Geometry check sheet. Reference: the model listing, model coordinates, mm. A direction names the side the tool comes from. Round coordinates to 2 decimals unless told otherwise and drop trailing zeros. Order: outer loops, then holes, each group sorted by start corner. A loop starts at its lowest first (then second) coordinate and runs counter-clockwise, first axis right, second up.
(1) Sectioned sample at A-A (y = 8). Record the boundary of the cut face in (x, z), plus the area to 3 significant figures.
(2) Go/stop test with flat-tipped pins: pin 1 (5 mm diameter, centred on x = -86, y = 2.5, fed in from -Z); pin 2 (4.5 mm diameter, centred on x = 4.5, y = 6.5, fed in from -Z); pin 3 (6 mm diameter, centred on x = -130.5, y = 4, fed in from -Z); pin 4 (0.6 mm diameter, centred on x = -24, y = 0.5, fed in from +Z). Record where each tip stops, or that it passes through.
(3) Release check for a two-part mould opening along X. For faces 1 (the face through (-104.89, 6.45, -107.23)), 2 (the face through (-2.734, 10.887, -2.675)), 3 (the face through (4, 8, -91)) record: +X half, -X half, draft (parallel to the pull), parting line (faces both ways), or undercut.
(4) Material ranges on line 1 along Y through (x, z) = (-51.5, -73.5); line 2 along X through (y, z) = (2.75, -13.5); line 3 along Z through (x, y) = (-60.5, 7.25), recorded low to high.
(5) Set-up check for faces 4 (the face through (-90, 8, -5)), 5 (the face through (-103.064, 0.838, -100.822)), 6 (the face through (-1, 11.8, -2)), 7 (the face through (5, 5.65, -95)), 8 (the face through (4, 8, -99.277)): record each of +Z, -Z, +X, -X, +Y, -Y from which the full face is reachable in a straight line by a thin tool's end or side.
from build123d import *

# Parameters (mm, degrees)
SKETCH1_R           = 150
BOSS_EXTRUDE3_DEPTH = 10
CUT_EXTRUDE2_DEPTH  = 10
BOSS_EXTRUDE4_DEPTH = 1.8
SKETCH6_W           = 3
SKETCH6_H           = 7
BOSS_EXTRUDE5_DEPTH = 2
SKETCH7_W           = 7
SKETCH7_H           = 3
BOSS_EXTRUDE6_DEPTH = 2
SKETCH8_W           = 10
SKETCH8_H           = 10
CUT_EXTRUDE3_DEPTH  = 5
SKETCH9_W           = 9.193751657
SKETCH9_H           = 8.277315045
BOSS_EXTRUDE7_DEPTH = 4.35
CHAMFER1_SIZE       = 1
CUT_EXTRUDE4_DEPTH  = 1.7
CUT_EXTRUDE5_DEPTH  = 0.8
FILLET1_R           = 3
FILLET2_R           = 1.4


with BuildPart() as part:
    # Sketch1 → Boss-Extrude3 (new body)
    with BuildSketch(Plane(origin=(0, 0, 0), x_dir=(1, 0, 0), z_dir=(0, 1, 0))):
        with Locations(Location((0, 0, 0), (0, 0, 270))):
            Circle(SKETCH1_R)
    extrude(amount=BOSS_EXTRUDE3_DEPTH)

    # Sketch4 → Cut-Extrude2 (cut)
    with BuildSketch(Plane(origin=(0, 10, 0), x_dir=(1, 0, 0), z_dir=(0, 1, 0))):
        Polygon((0, 0), (0, 162.329653064), (183.678217859, 162.329653064), (183.678217859, -176.427761891), (-217.916482153, -176.427761891), (-217.916482153, 0), align=None)
    extrude(amount=-CUT_EXTRUDE2_DEPTH, mode=Mode.SUBTRACT)

    # Sketch5 → Boss-Extrude4 (add)
    with BuildSketch(Plane(origin=(0, 10, 0), x_dir=(1, 0, 0), z_dir=(0, 1, 0))):
        with BuildLine():
            Line((0, 3.825), (0, 0))
            Line((0, 0), (-3.825, 0))
            ThreePointArc((-3.825, 0), (-2.704683438, 2.704683438), (0, 3.825))
        make_face()
    extrude(amount=BOSS_EXTRUDE4_DEPTH)

    # Sketch6 → Boss-Extrude5 (add)
    with BuildSketch(Plane(origin=(0, 10, 0), x_dir=(1, 0, 0), z_dir=(0, 1, 0))):
        with Locations((-28.5, 3.5)):
            Rectangle(SKETCH6_W, SKETCH6_H)
    extrude(amount=BOSS_EXTRUDE5_DEPTH)

    # Sketch7 → Boss-Extrude6 (add)
    with BuildSketch(Plane(origin=(0, 10, 0), x_dir=(1, 0, 0), z_dir=(0, 1, 0))):
        with Locations((-3.5, 28.5)):
            Rectangle(SKETCH7_W, SKETCH7_H)
    extrude(amount=BOSS_EXTRUDE6_DEPTH)

    # Sketch8 → Cut-Extrude3 (cut)
    with BuildSketch(Plane(origin=(0, 10, 0), x_dir=(1, 0, 0), z_dir=(0, 1, 0))):
        with Locations((-95, 5)):
            Rectangle(SKETCH8_W, SKETCH8_H)
    extrude(amount=-CUT_EXTRUDE3_DEPTH, mode=Mode.SUBTRACT)

    # Sketch9 → Boss-Extrude7 (add)
    with BuildSketch(Plane(origin=(0, 10, 0), x_dir=(1, 0, 0), z_dir=(0, 1, 0))):
        with Locations((4.596875828, 95.138657523)):
            Rectangle(SKETCH9_W, SKETCH9_H)
    extrude(amount=-BOSS_EXTRUDE7_DEPTH)

    # Chamfer1
    chamfer1_edges = [part.edges().sort_by_distance(p)[0] for p in [
        (9.193751657, 7.825, -99.277315045),
        (9.193751657, 7.825, -91),
    ]]
    chamfer(chamfer1_edges, length=CHAMFER1_SIZE)

    # Sketch10 → Cut-Extrude4 (cut)
    with BuildSketch(Plane.XZ):
        with BuildLine():
            Line((-140.926536809, 0), (-144.178447036, 0))
            ThreePointArc((-144.178447036, 0), (-101.9495576, -101.9495576), (0, -144.178447036))
            Line((0, -144.178447036), (0, -140.926536809))
            ThreePointArc((0, -140.926536809), (-99.650109827, -99.650109827), (-140.926536809, 0))
        make_face()
    extrude(amount=-CUT_EXTRUDE4_DEPTH, mode=Mode.SUBTRACT)

    # Sketch11 → Cut-Extrude5 (cut)
    with BuildSketch(Plane(origin=(0, 0, 0), x_dir=(-1, 0, 0), z_dir=(0, -1, 0))):
        Polygon((47, 0), (50, 0), (50, 50), (0, 50), (0, 47), (47, 47), align=None)
    extrude(amount=-CUT_EXTRUDE5_DEPTH, mode=Mode.SUBTRACT)

    # Fillet1
    fillet1_edges = [part.edges().sort_by_distance(p)[0] for p in [
        (-106.066017178, 0, -106.066017178),
    ]]
    fillet(fillet1_edges, radius=FILLET1_R)

    # Fillet2
    fillet2_edges = [part.edges().sort_by_distance(p)[0] for p in [
        (0, 5.65, -95.138657523),
    ]]
    fillet(fillet2_edges, radius=FILLET2_R)


solid = part.part
Answer below:
1. outline: (-150, 0) arc R150 ccw to (0, -150) - (0, -99.28) - (8.19, -99.28) - (9.19, -98.28) - (9.19, -92) - (8.19, -91) - (0, -91) - (0, 0) - (-90, 0) - (-90, -10) - (-100, -10) - (-100, 0) - close
1. area: 17,600 mm2
2. pin 1: stops at z = -124.59
2. pin 2: stops at z = -99.28
2. pin 3: stops at z = -79.02
2. pin 4: stops at z = 0
3. face 1: -X half
3. face 2: undercut
3. face 3: draft
4. line 1: y = 0 to 10
4. line 2: x = -149.38 to 0
4. line 3: z = -137.26 to 0
5. face 4: +Z, +Y
5. face 5: -Y
5. face 6: +Z, +X, +Y
5. face 7: +Z, -Z, +X, -Y
5. face 8: -Z, +X, +Y, -Y
